```python
from build123d import *

# Parameters (mm, degrees)
F1_DEPTH = 5
F2_R     = 2
F3_R     = 1


with BuildPart() as f1:
    # F0 (on Top) → F1 (new body)
    with BuildSketch(Plane.XY):
        with BuildLine():
            Line((-60.498083, 0), (-55.498083, 0))
            Line((-55.498083, 0), (-55.498083, 33.258991))
            ThreePointArc((-55.498083, 33.258991), (-54.047202, 38.446723), (-50.115569, 42.129099))
            Line((-50.115569, 42.129099), (-27.940299, 53.672814))
            Line((-27.940299, 53.672814), (-30.249042, 58.107868))
            Line((-30.249042, 58.107868), (-52.424312, 46.564153))
            ThreePointArc((-52.424312, 46.564153), (-58.321761, 41.040589), (-60.498083, 33.258991))
            Line((-60.498083, 33.258991), (-60.498083, 0))
        make_face()
    extrude(amount=F1_DEPTH)

    # F2
    f2_edges = [f1.edges().sort_by_distance(p)[0] for p in [
        (-55.498083, 16.629495, 0),
    ]]
    fillet(f2_edges, radius=F2_R)

    # F3
    f3_edges = [f1.edges().sort_by_distance(p)[0] for p in [
        (-60.498083, 16.629495, 0),
    ]]
    fillet(f3_edges, radius=F3_R)


solid = f1.part
```
The model under review builds one solid part; all positions refer to its coordinate system, in mm. A direction names the side the tool comes from. Coordinates: 2 decimals unless noted, no trailing zeros. Write each loop counter-clockwise with the first axis right and the second up, starting at its lowest first coordinate (ties: lowest second). Pieces come first, ordered by that corner, then holes.
1) To check wall thickness, follow probe 1 along X at (y, z) = (28, 2.65); probe 2 along X at (y, z) = (14, 0.6); probe 3 along Y at (x, z) = (-37, 0.5). State the ranges of each line that lie inside material, in increasing order.
2) Machinability: for faces 1 (the face through (-58.26, 41.14, 2.97)), 2 (the face through (-56.07, 16.86, 0.6)), 3 (the face through (-55.498, 16, 3)), which of the approach directions +Z, -Z, +X, -X, +Y, -Y give a long, thin tool a straight path to every point of the face, cutting with its end or side? Answer none if there is none.
3) We need section A-A on z = 2.95. State the section outline as (x, y) points.
4) The part is to be moulded in two halves that separate along Y. For faces 4 (the face through (-58, 0, 2)), 5 (the face through (-41.353, 51.988, 0.285)), 6 (the face through (-56, 31, 5)), say which applies: pulls with the +Y half, pulls with the -Y half, needs draft (parallel to the pull), parting line crosses it, or undercut.
5) We need section B-B on y = 6.5. State the section outline as (x, z) points, then the cut area to 3 significant figures.
6) Clearance check with flat-ended pins moving along their axes: pin 1 Ø4 at (x, y) = (-55, 21) entering from -Z; pin 2 Ø2 at (x, z) = (-48, 3) entering from +Y; pin 3 Ø2.5 at (y, z) = (8.5, 4) entering from +X. State where each tip first meets the part, or that it passes through.
Answer list:
1. probe 1: x = -60.5 to -55.5
1. probe 2: x = -60.41 to -56.07
1. probe 3: y = 49.72 to 54.44
2. face 1: +Z, -Z, -X, +Y
2. face 2: -Z, +X, -Y
2. face 3: +Z, -Z, +X, -Y
3. outline: (-60.5, 0) - (-55.5, 0) - (-55.5, 33.26) arc R10 cw to (-50.12, 42.13) - (-27.94, 53.67) - (-30.25, 58.11) - (-52.42, 46.56) arc R15 ccw to (-60.5, 33.26) - close
4. face 4: pulls with the -Y half
4. face 5: pulls with the +Y half
4. face 6: needs draft
5. outline: (-60.5, 1) arc R1 ccw to (-59.5, 0) - (-57.5, 0) arc R2 ccw to (-55.5, 2) - (-55.5, 5) - (-60.5, 5) - close
5. area: 23.9 mm2
6. pin 1: stops at z = 0.06
6. pin 2: stops at y = 49.39
6. pin 3: stops at x = -55.5
